```python
from build123d import *

# Parameters (mm, degrees)
BOSS_EXTRUDE1_DEPTH      = 42.5
BOSS_EXTRUDE1_DEPTH_BACK = 15
SKETCH1_W                = 40
SKETCH1_H                = 65
SKETCH3_W                = 22.5
SKETCH3_H                = 50
CUT_EXTRUDE2_DEPTH       = 30
SKETCH4_R                = 4.5
CUT_EXTRUDE3_DEPTH       = 10
SKETCH6_W                = 40
SKETCH6_H                = 65
CUT_EXTRUDE4_DEPTH       = 5
SKETCH7_R                = 3.1
CUT_EXTRUDE5_DEPTH       = 10
SKETCH8_W                = 52.5
SKETCH8_H                = 65
CUT_EXTRUDE6_DEPTH       = 5
SKETCH9_W                = 12.5
SKETCH9_H                = 12.5
SKETCH9_R                = 2.6
BOSS_EXTRUDE2_DEPTH      = 5
BOSS_EXTRUDE3_START      = 5
SKETCH10_R               = 3.1
BOSS_EXTRUDE3_DEPTH      = 5
SKETCH11_R               = 1.6
CUT_EXTRUDE7_DEPTH       = 87.240941553
CUT_EXTRUDE8_DEPTH       = 11.5
CUT_EXTRUDE8_DEPTH_BACK  = 11.5
SKETCH12_W               = 30
SKETCH12_H               = 50
CUT_EXTRUDE9_DEPTH       = 30
CUT_EXTRUDE10_DEPTH      = 15
CUT_EXTRUDE11_START      = -13
SKETCH15_R               = 17
SKETCH15_R_2             = 4.5
CUT_EXTRUDE11_DEPTH      = 13
CHAMFER1_SIZE            = 1
SKETCH16_W               = 9.25
SKETCH16_H               = 10
CUT_EXTRUDE12_DEPTH      = 2
SKETCH17_R               = 2.1
BOSS_EXTRUDE4_DEPTH      = 5
CHAMFER2_SIZE            = 5
CHAMFER3_SIZE            = 5
CHAMFER4_SIZE            = 5
SKETCH18_W               = 3
SKETCH18_H               = 15
CUT_EXTRUDE13_DEPTH      = 40.75
SKETCH20_R               = 1.2
BOSS_EXTRUDE5_DEPTH      = 5


with BuildPart() as part:
    # Sketch1 → Boss-Extrude1 (new, two sides: drawn at the far end of the back side and taken through both)
    with BuildSketch(Plane.XY.offset(-BOSS_EXTRUDE1_DEPTH_BACK)):
        with Locations((20, 32.5)):
            Rectangle(SKETCH1_W, SKETCH1_H)
    extrude(amount=BOSS_EXTRUDE1_DEPTH + BOSS_EXTRUDE1_DEPTH_BACK)

    # Sketch3 → Cut-Extrude2 (cut)
    with BuildSketch(Plane(origin=(40, 0, 0), x_dir=(0, 0, -1), z_dir=(1, 0, 0))):
        with Locations((-11.25, 40)):
            Rectangle(SKETCH3_W, SKETCH3_H)
    extrude(amount=-CUT_EXTRUDE2_DEPTH, mode=Mode.SUBTRACT)

    # Sketch4 → Cut-Extrude3 (cut)
    with BuildSketch(Plane(origin=(10, 0, 0), x_dir=(0, 0, -1), z_dir=(1, 0, 0))):
        with Locations((-11.25, 26.5)):
            Circle(SKETCH4_R)
    extrude(amount=-CUT_EXTRUDE3_DEPTH, mode=Mode.SUBTRACT)

    # Sketch6 → Cut-Extrude4 (cut)
    with BuildSketch(Plane.XY.offset(42.5)):
        with Locations((20, 32.5)):
            Rectangle(SKETCH6_W, SKETCH6_H)
    extrude(amount=-CUT_EXTRUDE4_DEPTH, mode=Mode.SUBTRACT)

    # Sketch7 → Cut-Extrude5 (cut)
    with BuildSketch(Plane.XZ):
        with Locations(Location((28, 25.5, 0), (0, 0, 270))):
            Circle(SKETCH7_R)
        with Locations(Location((28, -3, 0), (0, 0, 270))):
            Circle(SKETCH7_R)
    extrude(amount=-CUT_EXTRUDE5_DEPTH, mode=Mode.SUBTRACT)

    # Sketch8 → Cut-Extrude6 (cut)
    with BuildSketch(Plane.ZY):
        with Locations((11.25, 32.5)):
            Rectangle(SKETCH8_W, SKETCH8_H)
    extrude(amount=-CUT_EXTRUDE6_DEPTH, mode=Mode.SUBTRACT)

    # Sketch9 → Boss-Extrude2 (add)
    # profile 1 of 4: a face of its own
    with BuildSketch(Plane.XY.offset(37.5)):
        with Locations((-1.25, 58.75)):
            Rectangle(SKETCH9_W, SKETCH9_H)
        with Locations((-1.25, 58.75)):
            Circle(SKETCH9_R, mode=Mode.SUBTRACT)
    # profile 2 of 4: a face of its own
    with BuildSketch(Plane.XY.offset(37.5)):
        with Locations((46.25, 58.75)):
            Rectangle(SKETCH9_W, SKETCH9_H)
        with Locations(Location((46.25, 58.75, 0), (0, 0, 180))):
            Circle(SKETCH9_R, mode=Mode.SUBTRACT)
    # profile 3 of 4: a face of its own
    with BuildSketch(Plane.XY.offset(37.5)):
        with Locations((46.25, 6.25)):
            Rectangle(SKETCH9_W, SKETCH9_H)
        with Locations((46.25, 6.25)):
            Circle(SKETCH9_R, mode=Mode.SUBTRACT)
    # profile 4 of 4: a face of its own
    with BuildSketch(Plane.XY.offset(37.5)):
        with Locations((-1.25, 6.25)):
            Rectangle(SKETCH9_W, SKETCH9_H)
        with Locations(Location((-1.25, 6.25, 0), (0, 0, 180))):
            Circle(SKETCH9_R, mode=Mode.SUBTRACT)
    extrude(amount=-BOSS_EXTRUDE2_DEPTH)

    # Sketch10 → Boss-Extrude3 (add)
    with BuildSketch(Plane.XZ.offset(BOSS_EXTRUDE3_START)):
        Polygon((40, 32.5), (40, 37.5), (5, 37.5), (5, -15), (40, -15), align=None)
        with Locations(Location((28, 25.5, 0), (0, 0, 270))):
            Circle(SKETCH10_R, mode=Mode.SUBTRACT)
        with Locations(Location((28, -3, 0), (0, 0, 270))):
            Circle(SKETCH10_R, mode=Mode.SUBTRACT)
    extrude(amount=-BOSS_EXTRUDE3_DEPTH)

    # Sketch11 → Cut-Extrude7 (cut, through all)
    with BuildSketch(Plane(origin=(10, 0, 0), x_dir=(0, 0, -1), z_dir=(1, 0, 0))):
        with Locations((-2.5, 47)):
            Circle(SKETCH11_R)
        with Locations((-20, 47)):
            Circle(SKETCH11_R)
    extrude(amount=-CUT_EXTRUDE7_DEPTH, mode=Mode.SUBTRACT)

    # Sketch12 → Cut-Extrude8 (cut, two sides: drawn at the far end of the back side and taken through both)
    with BuildSketch(Plane(origin=(0, 0, 11.25), x_dir=(-1, 0, 0), z_dir=(0, 0, -1)).offset(-CUT_EXTRUDE8_DEPTH_BACK)):
        with Locations((-25, 40)):
            Rectangle(SKETCH12_W, SKETCH12_H)
    extrude(amount=CUT_EXTRUDE8_DEPTH + CUT_EXTRUDE8_DEPTH_BACK, mode=Mode.SUBTRACT)

    # Sketch13 → Cut-Extrude9 (cut)
    with BuildSketch(Plane(origin=(40, 0, 0), x_dir=(0, 0, -1), z_dir=(1, 0, 0))):
        Polygon((-11.25, 15), (-8.25, 15), (-8.25, 9), (-14.25, 9), (-14.25, 15), align=None)
    extrude(amount=-CUT_EXTRUDE9_DEPTH, mode=Mode.SUBTRACT)

    # Sketch14 → Cut-Extrude10 (cut)
    with BuildSketch(Plane(origin=(0, 65, 0), x_dir=(1, 0, 0), z_dir=(0, 1, 0))):
        Polygon((5, -11.25), (5, -8.25), (10, -8.25), (10, -14.25), (5, -14.25), align=None)
    extrude(amount=-CUT_EXTRUDE10_DEPTH, mode=Mode.SUBTRACT)

    # Sketch15 → Cut-Extrude11 (cut)
    # profile 1 of 2: a face of its own
    with BuildSketch(Plane.ZY.offset(-5).offset(CUT_EXTRUDE11_START)):
        with Locations((11.25, 26.5)):
            Circle(SKETCH15_R)
        with Locations((11.25, 26.5)):
            Circle(SKETCH15_R_2, mode=Mode.SUBTRACT)
    # profile 2 of 2: a face of its own
    with BuildSketch(Plane.ZY.offset(-5).offset(CUT_EXTRUDE11_START)):
        with BuildLine():
            Line((-5.75, 26.5), (-5.75, -5))
            Line((-5.75, -5), (28.25, -5))
            Line((28.25, -5), (28.25, 26.5))
            ThreePointArc((28.25, 26.5), (11.25, 9.5), (-5.75, 26.5))
        make_face()
    extrude(amount=CUT_EXTRUDE11_DEPTH, mode=Mode.SUBTRACT)

    # Chamfer1
    chamfer1_edges = [part.edges().sort_by_distance(p)[0] for p in [
        (5, 10.75, -5.75),
        (5, 43.5, 11.25),
        (5, 10.75, 28.25),
    ]]
    chamfer(chamfer1_edges, length=CHAMFER1_SIZE)

    # Sketch16 → Cut-Extrude12 (cut)
    with BuildSketch(Plane.ZY.offset(-5)):
        with Locations((-10.375, 0)):
            Rectangle(SKETCH16_W, SKETCH16_H)
    extrude(amount=-CUT_EXTRUDE12_DEPTH, mode=Mode.SUBTRACT)

    # Sketch17 → Boss-Extrude4 (add)
    # profile 1 of 3: a face of its own
    with BuildSketch(Plane(origin=(69.218616892, 6.6, 8.180920591), x_dir=(-1, 0, 0), z_dir=(0, -1, 0))):
        Polygon((51.218616892, 7.230920591), (51.218616892, 2.230920591), (56.218616892, 2.230920591), align=None)
    # profile 2 of 3: a face of its own
    with BuildSketch(Plane(origin=(69.218616892, 6.6, 8.180920591), x_dir=(-1, 0, 0), z_dir=(0, -1, 0))):
        Polygon((56.218616892, -9.769079409), (51.218616892, -9.769079409), (51.218616892, -14.569079409), align=None)
    # profile 3 of 3: a face of its own
    with BuildSketch(Plane(origin=(69.218616892, 6.6, 8.180920591), x_dir=(-1, 0, 0), z_dir=(0, -1, 0))):
        Polygon((56.218616892, 2.230920591), (51.218616892, 2.230920591), (51.218616892, -9.769079409), (56.218616892, -9.769079409), (82.218616892, -9.769079409), (82.218616892, 2.230920591), align=None)
        with Locations(Location((56.721116892, -3.069079409, 0), (0, 0, 180))):
            Circle(SKETCH17_R, mode=Mode.SUBTRACT)
        with Locations(Location((76.541116892, -3.069079409, 0), (0, 0, 180))):
            Circle(SKETCH17_R, mode=Mode.SUBTRACT)
    extrude(amount=BOSS_EXTRUDE4_DEPTH)

    # Chamfer2
    chamfer2_edges = [part.edges().sort_by_distance(p)[0] for p in [
        (40, -5, 11.25),
    ]]
    chamfer(chamfer2_edges, length=CHAMFER2_SIZE)

    # Chamfer3
    chamfer3_edges = [part.edges().sort_by_distance(p)[0] for p in [
        (40, 52.5, 35),
        (40, 12.5, 35),
    ]]
    chamfer(chamfer3_edges, length=CHAMFER3_SIZE)

    # Chamfer4
    chamfer4_edges = [part.edges().sort_by_distance(p)[0] for p in [
        (5, 12.5, 35),
        (5, 52.5, 35),
    ]]
    chamfer(chamfer4_edges, length=CHAMFER4_SIZE)

    # Sketch18 → Cut-Extrude13 (cut)
    with BuildSketch(Plane(origin=(0, 0, -15), x_dir=(-1, 0, 0), z_dir=(0, 0, -1))):
        with Locations((-31, 49.5)):
            Rectangle(SKETCH18_W, SKETCH18_H)
    extrude(amount=-CUT_EXTRUDE13_DEPTH, mode=Mode.SUBTRACT)

    # Sketch20 → Boss-Extrude5 (add)
    with BuildSketch(Plane.ZY.offset(-17)):
        Polygon((-15, -3.25), (-35, -3.2), (-35, 6.7), (-15, 6.7), align=None)
        with Locations((-29.75, 3.9)):
            Circle(SKETCH20_R, mode=Mode.SUBTRACT)
        with Locations((-20.15, 3.9)):
            Circle(SKETCH20_R, mode=Mode.SUBTRACT)
    extrude(amount=BOSS_EXTRUDE5_DEPTH)


solid = part.part
```
Build history of the part. All positions in model axes, mm. A direction names the side the tool comes from. Round coordinates to 2 decimals unless told otherwise and drop trailing zeros. Write each loop counter-clockwise with the first axis right and the second up, starting at its lowest first coordinate (ties: lowest second). Pieces come first, ordered by that corner, then holes. Notation, with made-up numbers: (48, 45) - (76, 45) arc R33 cw to (76, 78) - close; hole circle Ø3 at (36.5, 66). An arc over 180 degrees is marked (long way). Answer as CSV lines item,"result".
Q1. Cut at A-A (x = 46.25). Write the cut outline in (y, z).
Report:
outline,"(0, 32.5) - (3.65, 32.5) - (3.65, 37.5) - (0, 37.5) - close; (8.85, 32.5) - (12.5, 32.5) - (12.5, 37.5) - (8.85, 37.5) - close; (52.5, 32.5) - (56.15, 32.5) - (56.15, 37.5) - (52.5, 37.5) - close; (61.35, 32.5) - (65, 32.5) - (65, 37.5) - (61.35, 37.5) - close"
Q2. Drill centre lines: probe 1 along Y at (x, z) = (-1.25, 33.7); probe 2 along Z at (x, y) = (13.5, 22); probe 3 along Y at (x, z) = (14.6, -20.15). Where is each one in solid material? Low to high. Write a range as [from, to].
Report:
probe 1,"y = [0, 3.65], [8.85, 12.5], [52.5, 56.15], [61.35, 65]"
probe 2,"z = [-15, -5.75], [28.25, 37.5]"
probe 3,"y = [-3.24, 2.7], [5.1, 6.7]"
Q3. Drop flat-ended pins along their axis: pin 1 (4 mm diameter, centred on x = -1.5, z = 36, fed in from -Y); pin 2 (2.5 mm diameter, centred on x = 15, z = -21.5, fed in from +Y); pin 3 (4 mm diameter, centred on x = 46.25, y = 58.75, fed in from +Z); pin 4 (4 mm diameter, centred on x = 7, y = 54, fed in from -Z). Give the stop position or say it passes through.
Report:
pin 1,"stops at y = 0"
pin 2,"stops at y = 6.7"
pin 3,"passes through"
pin 4,"stops at z = -15"
Q4. Cut at D-D (z = 20). State how many separate pieces and enclosed holes the cut face has, and give its area (3 significant figures).
Report:
separate pieces,"3"
enclosed holes,"0"
area,"545 mm^2"
Q5. Cut at C-C (x = 36). Write the cut outline in (y, z).
Report:
outline,"(-4, -15) - (65, -15) - (65, -0.25) - (15, -0.25) - (15, 8.25) - (9, 8.25) - (9, 14.25) - (15, 14.25) - (15, 22.75) - (65, 22.75) - (65, 37.5) - (-4, 37.5) - close"
Q6. Tool access for faces 4 (the flat face through (29, 15, 4)), 5 (the flat face through (15.465, 4.135, 3.485)), 6 (the flat face through (-1, 0, 35)), 7 (the flat face through (0, 4, 5.95)): list every direction of +Z, -Z, +X, -X, +Y, -Y with a clear straight run to the whole face (end or side of a thin tool).
Report:
face 4,"+X, -X, +Y"
face 5,"-X, +Y, -Y"
face 6,"+Z, -Z, -X, -Y"
face 7,"-X, -Y"
Q7. Cut at B-B (z = -20.15). Write the cut outline in (x, y), and give its area (3 significant figures).
Report:
outline,"(12, -3.24) - (17, -3.24) - (17, 2.7) - (12, 2.7) - close; (12, 5.1) - (17, 5.1) - (17, 6.7) - (12, 6.7) - close"
area,"37.7 mm^2"
Q8. Pull direction Y, two halves, no side cores. Call faces 1 (the cylindrical face through (7.54, 45.58, 19.26)), 2 (the flat face through (12, 11, -5.75)), 3 (the flat face through (29, 15, 19)): +Y half, -Y half, draft (parallel to the pull), parting line (faces both ways), or undercut.
Report:
face 1,"undercut"
face 2,"draft"
face 3,"+Y half"
